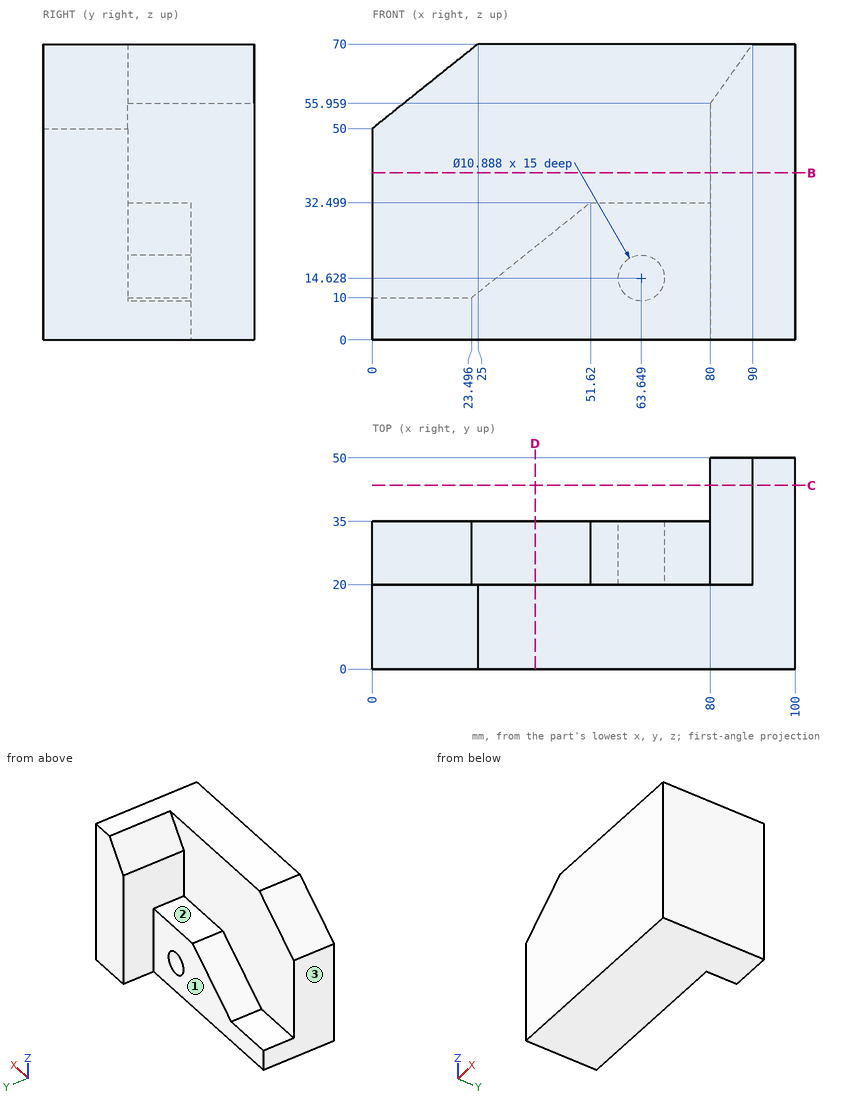
Can you work these out from the drawing? Everything is in mm from the part's minimum corner. A direction names the side the tool comes from. Give positions to 0.01 mm unless a question says otherwise; leave off trailing zeros. Order: outer loops, then holes, each group sorted by start corner. A loop starts at its lowest first (then second) coordinate and runs counter-clockwise, first axis right, second up.
Item 1: If we section it at B-B, the plane z = 39.5: Write out the boundary of the cut face in (x, y).
Item 2: I'm going to push flat-ended pins straight in: pin 1 (5 mm diameter, centred on x = 84.5, y = 38.5, fed in from +Z); pin 2 (6.5 mm diameter, centred on x = 63.65, z = 14.63, fed in from +Y); pin 3 (24 mm diameter, centred on y = 33.5, z = 38.5, fed in from -X). Where does each tip first touch, or does it pass through?
Item 3: If we section it at D-D, the plane x = 38.5: Write out the boundary of the cut face in (y, z), plus the area to 3 significant figures.
Item 4: If we section it at C-C, the plane y = 43.5: Write out the boundary of the cut face in (x, z), plus the area to 3 significant figures.
Item 5: I need wall thicknesses on line 1 (Y direction, x = 35, z = 43.5); line 2 (X direction, y = 37, z = 20); line 3 (X direction, y = 13.5, z = 66). Which ranges of each line are inside material? Lowest first, please.
Item 6: For the marked faces 1, 2 and 3, which set-ups out of +Z, -Z, +X, -X, +Y, -Y let a thin tool reach every point of the face, with its end or its side?
Values:
1. outline: (0, 0) - (100, 0) - (100, 50) - (80, 50) - (80, 20) - (0, 20) - close
2. pin 1: stops at z = 65.79
2. pin 2: stops at y = 20
2. pin 3: stops at x = 44.12
3. outline: (0, 0) - (35, 0) - (35, 22) - (20, 22) - (20, 70) - (0, 70) - close
3. area: 1,730 mm2
4. outline: (80, 0) - (100, 0) - (100, 70) - (90, 70) - (80, 55.96) - close
4. area: 1,330 mm2
5. line 1: y = 0 to 20
5. line 2: x = 80 to 100
5. line 3: x = 20 to 100
6. face 1: +Z, -Z, -X, +Y
6. face 2: +Z, -X, +Y
6. face 3: +Z, -Z, -X, +Y, -Y
